from build123d import *

# Parameters (mm, degrees)
SKETCH1_W                   = 25.4
SKETCH1_H                   = 25.4
SKETCH1_W_2                 = 22.225
SKETCH1_H_2                 = 22.225
BOSS_EXTRUDE1_DEPTH         = 254
F_22_0_157_DIAMETER_HOLE1_D = 3.9878
LPATTERN1_COUNT             = 20
LPATTERN1_PITCH             = 12.7
F_22_0_157_DIAMETER_HOLE2_D = 3.9878
LPATTERN2_COUNT             = 20
LPATTERN2_PITCH             = 12.7


with BuildPart() as part:
    # Sketch1 → Boss-Extrude1 (new body)
    with BuildSketch(Plane(origin=(0, 0, 0), x_dir=(1, 0, 0), z_dir=(0, 1, 0))):
        Rectangle(SKETCH1_W, SKETCH1_H)
        Rectangle(SKETCH1_W_2, SKETCH1_H_2, mode=Mode.SUBTRACT)
    extrude(amount=BOSS_EXTRUDE1_DEPTH)

    # #22 (0.157) Diameter Hole1 (through all)
    with Locations(Plane.XY.offset(12.7)):
        with Locations((0, 12.7)):
            f_22_0_157_diameter_hole1 = Hole(F_22_0_157_DIAMETER_HOLE1_D / 2)

    # LPattern1: #22 (0.157) Diameter Hole1 ×20
    with Locations(*[(0, i * LPATTERN1_PITCH, 0) for i in range(1, LPATTERN1_COUNT)]):
        add(f_22_0_157_diameter_hole1, mode=Mode.SUBTRACT)

    # #22 (0.157) Diameter Hole2 (through all)
    with Locations(Plane(origin=(12.7, 0, 0), x_dir=(0, 0, -1), z_dir=(1, 0, 0))):
        with Locations((0, 12.7)):
            f_22_0_157_diameter_hole2 = Hole(F_22_0_157_DIAMETER_HOLE2_D / 2)

    # LPattern2: #22 (0.157) Diameter Hole2 ×20
    with Locations(*[(0, i * LPATTERN2_PITCH, 0) for i in range(1, LPATTERN2_COUNT)]):
        add(f_22_0_157_diameter_hole2, mode=Mode.SUBTRACT)


solid = part.part
Part model, mm, in its own coordinate system. A direction names the side the tool comes from. Coordinates: 2 decimals unless noted, no trailing zeros. Order: outer loops, then holes, each group sorted by start corner. A loop starts at its lowest first (then second) coordinate and runs counter-clockwise, first axis right, second up. Notation, with made-up numbers: (-2.5, 57) - (43.5, 57) arc R10 ccw to (43.5, 70) - close; hole circle Ø9 at (-38, -35.75). An arc over 180 degrees is marked (long way). Use CSV: the item, a comma, the result in double quotes.
Item 1: Saw through at A-A on z = 6.25. Give the cut face in (x, y).
Solved:
outline,"(-12.7, 0) - (-11.11, 0) - (-11.11, 254) - (-12.7, 254) - close; (11.11, 0) - (12.7, 0) - (12.7, 254) - (11.11, 254) - close"
Item 2: Mould opens along Z. For faces 3 (the face through (-11.917, 205.177, -0.26)), 4 (the face through (-9.8, 254, -11.3)), 5 (the face through (11.895, 103.281, 1.072)) say: +Z half, -Z half, draft (parallel to the pull), parting line (faces both ways), or undercut.
Solved:
face 3,"undercut"
face 4,"draft"
face 5,"undercut"
Item 3: Probe probe 1 along X at (y, z) = (81.5, 2.25); probe 2 along X at (y, z) = (152.4, -12.1). List the from-to ranges inside material, lowest first.
Solved:
probe 1,"x = -12.7 to -11.11, 11.11 to 12.7"
probe 2,"x = -12.7 to -1.99, 1.99 to 12.7"
Item 4: 3-axis set-ups, long thin cutter, end or side, ignore diameter. For faces 1 (the face through (-3, 125, 11.112)), 2 (the face through (-11.917, 167.077, -0.26)): which of +Z, -Z, +X, -X, +Y, -Y reach the whole face in a straight line?
Solved:
face 1,"+Y, -Y"
face 2,"+X, -X"
Item 5: Saw through at B-B on y = 122.5. Give the cut face in (x, z).
Solved:
outline,"(-12.7, -12.7) - (12.7, -12.7) - (12.7, 12.7) - (-12.7, 12.7) - close; hole (-11.11, -11.11) - (11.11, -11.11) - (11.11, 11.11) - (-11.11, 11.11) - close"
Item 6: Drop a flat-ended pin along its axis: P1, Ø2.5, axis at x = 0, y = 139.7, coming from the +Z side. Give the stop position or say it passes through.
Solved:
P1,"passes through"
